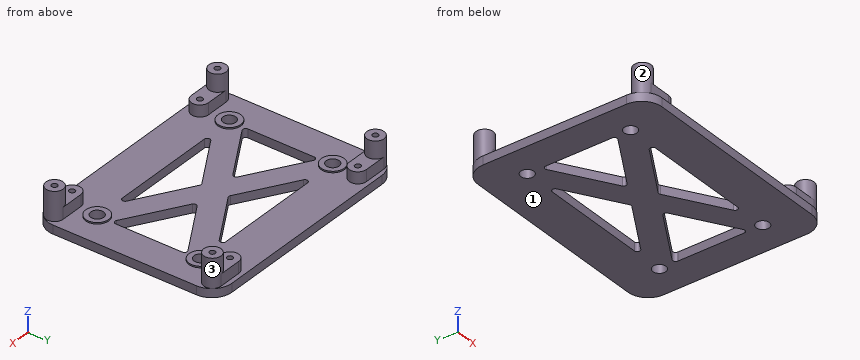
```python
from build123d import *

# Parameters (mm, degrees)
ESBO_O1_W                = 82
ESBO_O1_H                = 64
RESSALTO_EXTRUS_O1_DEPTH = 3
ESBO_O2_R                = 3
ESBO_O2_R_2              = 1
RESSALTO_EXTRUS_O2_DEPTH = 4
ESBO_O3_R                = 3
ESBO_O3_R_2              = 1
RESSALTO_EXTRUS_O3_DEPTH = 10
ESBO_O4_R                = 2.25
CORTE_EXTRUS_O1_DEPTH    = 53.962250707
RESSALTO_EXTRUS_O4_START = 0.5
ESBO_O5_R                = 4
ESBO_O5_R_2              = 2.25
RESSALTO_EXTRUS_O4_DEPTH = 0.5
FILETE1_R                = 7
CORTE_EXTRUS_O2_DEPTH    = 53.962250707
FILETE2_R                = 1
ESBO_O7_R                = 1
RESSALTO_EXTRUS_O5_DEPTH = 4


with BuildPart() as part:
    # Esboço1 → Ressalto-extrusão1 (new body)
    with BuildSketch(Plane.XY):
        Rectangle(ESBO_O1_W, ESBO_O1_H)
    extrude(amount=RESSALTO_EXTRUS_O1_DEPTH)

    # Esboço2 → Ressalto-extrusão2 (add)
    # profile 1 of 4: a face of its own
    with BuildSketch(Plane.XY.offset(3)):
        with Locations(Location((-29, 27.5, 0), (0, 0, 180))):
            Circle(ESBO_O2_R)
        with Locations((-29, 27.5)):
            Circle(ESBO_O2_R_2, mode=Mode.SUBTRACT)
    # profile 2 of 4: a face of its own
    with BuildSketch(Plane.XY.offset(3)):
        with Locations(Location((-29, -27.5, 0), (0, 0, 180))):
            Circle(ESBO_O2_R)
        with Locations(Location((-29, -27.5, 0), (0, 0, 180))):
            Circle(ESBO_O2_R_2, mode=Mode.SUBTRACT)
    # profile 3 of 4: a face of its own
    with BuildSketch(Plane.XY.offset(3)):
        with Locations(Location((29, -27.5, 0), (0, 0, 180))):
            Circle(ESBO_O2_R)
        with Locations((29, -27.5)):
            Circle(ESBO_O2_R_2, mode=Mode.SUBTRACT)
    # profile 4 of 4: a face of its own
    with BuildSketch(Plane.XY.offset(3)):
        with Locations(Location((29, 27.5, 0), (0, 0, 180))):
            Circle(ESBO_O2_R)
        with Locations(Location((29, 27.5, 0), (0, 0, 180))):
            Circle(ESBO_O2_R_2, mode=Mode.SUBTRACT)
    extrude(amount=RESSALTO_EXTRUS_O2_DEPTH)

    # Esboço3 → Ressalto-extrusão3 (add)
    # profile 1 of 4: a face of its own
    with BuildSketch(Plane.XY.offset(3)):
        with Locations(Location((-37, 27.5, 0), (0, 0, 180))):
            Circle(ESBO_O3_R)
        with Locations((-37, 27.5)):
            Circle(ESBO_O3_R_2, mode=Mode.SUBTRACT)
    # profile 2 of 4: a face of its own
    with BuildSketch(Plane.XY.offset(3)):
        with Locations(Location((37, 27.5, 0), (0, 0, 180))):
            Circle(ESBO_O3_R)
        with Locations(Location((37, 27.5, 0), (0, 0, 180))):
            Circle(ESBO_O3_R_2, mode=Mode.SUBTRACT)
    # profile 3 of 4: a face of its own
    with BuildSketch(Plane.XY.offset(3)):
        with Locations(Location((37, -27.5, 0), (0, 0, 180))):
            Circle(ESBO_O3_R)
        with Locations((37, -27.5)):
            Circle(ESBO_O3_R_2, mode=Mode.SUBTRACT)
    # profile 4 of 4: a face of its own
    with BuildSketch(Plane.XY.offset(3)):
        with Locations(Location((-37, -27.5, 0), (0, 0, 180))):
            Circle(ESBO_O3_R)
        with Locations(Location((-37, -27.5, 0), (0, 0, 180))):
            Circle(ESBO_O3_R_2, mode=Mode.SUBTRACT)
    extrude(amount=RESSALTO_EXTRUS_O3_DEPTH)

    # Esboço4 → Corte-extrusão1 (cut, through all)
    with BuildSketch(Plane.XY.offset(3)):
        with Locations((-30, 18)):
            Circle(ESBO_O4_R)
        with Locations(Location((30, 18, 0), (0, 0, 180))):
            Circle(ESBO_O4_R)
        with Locations((30, -18)):
            Circle(ESBO_O4_R)
        with Locations(Location((-30, -18, 0), (0, 0, 180))):
            Circle(ESBO_O4_R)
    extrude(amount=-CORTE_EXTRUS_O1_DEPTH, mode=Mode.SUBTRACT)

    # Esboço5 → Ressalto-extrusão4 (add)
    # profile 1 of 4: a face of its own
    with BuildSketch(Plane.XY.offset(3).offset(RESSALTO_EXTRUS_O4_START)):
        with Locations(Location((-30, 18, 0), (0, 0, 180))):
            Circle(ESBO_O5_R)
        with Locations((-30, 18)):
            Circle(ESBO_O5_R_2, mode=Mode.SUBTRACT)
    # profile 2 of 4: a face of its own
    with BuildSketch(Plane.XY.offset(3).offset(RESSALTO_EXTRUS_O4_START)):
        with Locations(Location((30, 18, 0), (0, 0, 180))):
            Circle(ESBO_O5_R)
        with Locations(Location((30, 18, 0), (0, 0, 180))):
            Circle(ESBO_O5_R_2, mode=Mode.SUBTRACT)
    # profile 3 of 4: a face of its own
    with BuildSketch(Plane.XY.offset(3).offset(RESSALTO_EXTRUS_O4_START)):
        with Locations(Location((-30, -18, 0), (0, 0, 180))):
            Circle(ESBO_O5_R)
        with Locations(Location((-30, -18, 0), (0, 0, 180))):
            Circle(ESBO_O5_R_2, mode=Mode.SUBTRACT)
    # profile 4 of 4: a face of its own
    with BuildSketch(Plane.XY.offset(3).offset(RESSALTO_EXTRUS_O4_START)):
        with Locations(Location((30, -18, 0), (0, 0, 180))):
            Circle(ESBO_O5_R)
        with Locations((30, -18)):
            Circle(ESBO_O5_R_2, mode=Mode.SUBTRACT)
    extrude(amount=-RESSALTO_EXTRUS_O4_DEPTH)

    # Filete1
    filete1_edges = [part.edges().sort_by_distance(p)[0] for p in [
        (41, -32, 1.5),
        (-41, -32, 1.5),
        (-41, 32, 1.5),
        (41, 32, 1.5),
    ]]
    fillet(filete1_edges, radius=FILETE1_R)

    # Esboço6 → Corte-extrusão2 (cut, through all)
    with BuildSketch(Plane.XY.offset(3)):
        Polygon((-30, 13.335238484), (-7.774602526, 0), (-30, -13.335238484), align=None)
        Polygon((-22.225397474, -18), (0, -4.664761516), (22.225397474, -18), align=None)
        Polygon((-22.225397474, 18), (0, 4.664761516), (22.225397474, 18), align=None)
        Polygon((30, -13.335238484), (30, 13.335238484), (7.774602526, 0), align=None)
    extrude(amount=-CORTE_EXTRUS_O2_DEPTH, mode=Mode.SUBTRACT)

    # Filete2
    filete2_edges = [part.edges().sort_by_distance(p)[0] for p in [
        (22.225397474, -18, 1.5),
        (-22.225397474, -18, 1.5),
        (0, -4.664761516, 1.5),
        (-30, -13.335238484, 1.5),
        (-30, 13.335238484, 1.5),
        (-7.774602526, 0, 1.5),
        (30, -13.335238484, 1.5),
        (7.774602526, 0, 1.5),
        (30, 13.335238484, 1.5),
        (-22.225397474, 18, 1.5),
        (22.225397474, 18, 1.5),
        (0, 4.664761516, 1.5),
    ]]
    fillet(filete2_edges, radius=FILETE2_R)

    # Esboço7 → Ressalto-extrusão5 (add)
    # profile 1 of 4: a face of its own
    with BuildSketch(Plane.XY.offset(3)):
        with BuildLine():
            Line((-37, 30.5), (-29, 30.5))
            ThreePointArc((-29, 30.5), (-26, 27.5), (-29, 24.5))
            Line((-29, 24.5), (-37, 24.5))
            ThreePointArc((-37, 24.5), (-40, 27.5), (-37, 30.5))
        make_face()
        with Locations((-37, 27.5)):
            Circle(ESBO_O7_R, mode=Mode.SUBTRACT)
        with Locations((-29, 27.5)):
            Circle(ESBO_O7_R, mode=Mode.SUBTRACT)
    # profile 2 of 4: a face of its own
    with BuildSketch(Plane.XY.offset(3)):
        with BuildLine():
            Line((37, 24.5), (29, 24.5))
            ThreePointArc((29, 24.5), (26, 27.5), (29, 30.5))
            Line((29, 30.5), (37, 30.5))
            ThreePointArc((37, 30.5), (40, 27.5), (37, 24.5))
        make_face()
        with Locations(Location((29, 27.5, 0), (0, 0, 180))):
            Circle(ESBO_O7_R, mode=Mode.SUBTRACT)
        with Locations(Location((37, 27.5, 0), (0, 0, 180))):
            Circle(ESBO_O7_R, mode=Mode.SUBTRACT)
    # profile 3 of 4: a face of its own
    with BuildSketch(Plane.XY.offset(3)):
        with BuildLine():
            Line((37, -30.5), (29, -30.5))
            ThreePointArc((29, -30.5), (26, -27.5), (29, -24.5))
            Line((29, -24.5), (37, -24.5))
            ThreePointArc((37, -24.5), (40, -27.5), (37, -30.5))
        make_face()
        with Locations((37, -27.5)):
            Circle(ESBO_O7_R, mode=Mode.SUBTRACT)
        with Locations((29, -27.5)):
            Circle(ESBO_O7_R, mode=Mode.SUBTRACT)
    # profile 4 of 4: a face of its own
    with BuildSketch(Plane.XY.offset(3)):
        with BuildLine():
            Line((-37, -24.5), (-29, -24.5))
            ThreePointArc((-29, -24.5), (-26, -27.5), (-29, -30.5))
            Line((-29, -30.5), (-37, -30.5))
            ThreePointArc((-37, -30.5), (-40, -27.5), (-37, -24.5))
        make_face()
        with Locations(Location((-29, -27.5, 0), (0, 0, 180))):
            Circle(ESBO_O7_R, mode=Mode.SUBTRACT)
        with Locations(Location((-37, -27.5, 0), (0, 0, 180))):
            Circle(ESBO_O7_R, mode=Mode.SUBTRACT)
    extrude(amount=RESSALTO_EXTRUS_O5_DEPTH)


solid = part.part
```
For this review, take the finished solid that the model builds, in its own axes (mm). Face numbers are marked on the shaded views. Give positions to 0.01 mm unless a question says otherwise; leave off trailing zeros. Write each loop counter-clockwise with the first axis right and the second up, starting at its lowest first coordinate (ties: lowest second). Pieces come first, ordered by that corner, then holes. Notation, with made-up numbers: M 18,-9 L 46,-9 A12 ccw 46,13 Z; hole C -38,6.25 d4. An arc over 180 degrees is marked long. One line per item, written item: value.
1) The part is to be moulded in two halves that separate along Y. For the marked faces 1, 2 and 3, say which applies: +Y half, -Y half, draft (parallel to the pull), parting line (faces both ways), or undercut.
Results are:
face 1: draft
face 2: undercut
face 3: undercut
2) Take a section at B-B, the plane x = 16. Write out the cut boundary in (y, z), then the cut area to 3 significant figures.
Results are:
outline: M -32,0 L -18,0 L -18,3 L -32,3 Z; M -14.26,0 L -4.94,0 L -4.94,3 L -14.26,3 Z; M 4.94,0 L 14.26,0 L 14.26,3 L 4.94,3 Z; M 18,0 L 32,0 L 32,3 L 18,3 Z
area: 140 mm²
3) Take a section at D-D, the plane x = -6.5. Write out the cut boundary in (y, z).
Results are:
outline: M -32,0 L -18,0 L -18,3 L -32,3 Z; M -8.56,0 L 8.56,0 L 8.56,3 L -8.56,3 Z; M 18,0 L 32,0 L 32,3 L 18,3 Z
4) For P1, Ø2.5, axis at x = 28, y = 17.5, coming from the +Z side; P2, Ø5, axis at x = 31.5, y = 28.5, coming from the +Z side; P3, Ø2, axis at x = 35, z = 5.5, coming from the +Y side, all flat-tipped, find the tip position at first contact; note any pin that passes through.
Results are:
P1: stops at z = 3.5
P2: stops at z = 7
P3: stops at y = 30.5
5) For line 1 (Y direction, x = 29, z = 4); line 2 (X direction, y = -6, z = 2.25); line 3 (Z direction, x = -32, y = -25), list the stretches that pass through material, from the lowest coordinate up. Write a range as from..to.
Results are:
line 1: y = -30.5..-28.5, -26.5..-24.5, 24.5..26.5, 28.5..30.5
line 2: x = -41..-30, -17.77..-2.23, 2.23..17.77, 30..41
line 3: z = 0..7
6) Take a section at A-A, the plane z = 11. Write out the cut boundary in (x, y).
Results are:
outline: C -37,-27.5 d6; C -37,27.5 d6; C 37,-27.5 d6; C 37,27.5 d6; hole C -37,-27.5 d2; hole C -37,27.5 d2; hole C 37,-27.5 d2; hole C 37,27.5 d2
7) Take a section at C-C, the plane y = 10.5. Write out the cut boundary in (x, z).
Results are:
outline: M -41,0 L -30,0 L -30,3 L -41,3 Z; M -25.27,0 L -9.73,0 L -9.73,3 L -25.27,3 Z; M 9.73,0 L 25.27,0 L 25.27,3 L 9.73,3 Z; M 30,0 L 41,0 L 41,3 L 30,3 Z
